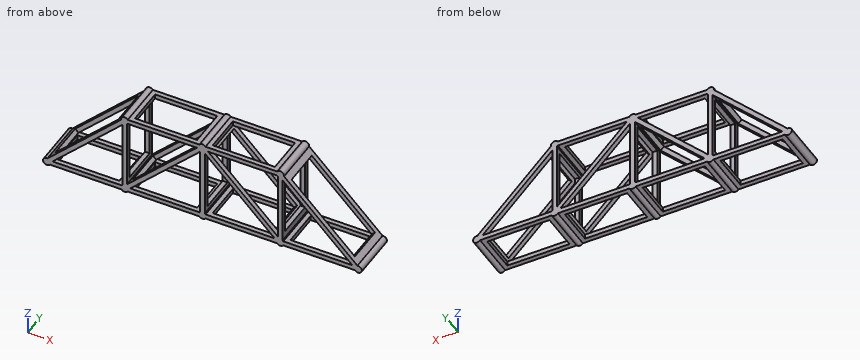
Autodesk Fusion 360 part; units mm, degrees
sketch "Sketch1" plane through (0, 0, 0) normal (0, 1, 0) x (1, 0, 0)
  circle A0 centre (-75, 0) radius 2.5
  line L0 (-75, 0) -> (25, 0) construction
  circle A1 centre (25, 0) radius 2.5
  line L1 (25, 0) -> (25, -50) construction
  line L2 (25, -50) -> (-25, -50) construction
  line L3 (-25, -50) -> (-75, 0) construction
  line L4 (25, -50) -> (-25, 0) construction
  line L5 (-25, -50) -> (-25, 0) construction
  circle A2 centre (-25, -50) radius 2.5
  circle A3 centre (25, -50) radius 2.5
  circle A4 centre (-25, 0) radius 2.5
  line L6 (-23.9393, -48.9393) -> (-73.9393, 1.0607)
  line L7 (-26.0607, -51.0607) -> (-76.0607, -1.0607)
  line L8 (25, -48.5) -> (-25, -48.5)
  line L9 (25, -51.5) -> (-25, -51.5)
  line L10 (23.5, 0) -> (23.5, -50)
  line L11 (26.5, 0) -> (26.5, -50)
  line L12 (23.9393, -51.0607) -> (-26.0607, -1.0607)
  line L13 (26.0607, -48.9393) -> (-23.9393, 1.0607)
  line L14 (-75, -1.5) -> (25, -1.5)
  line L15 (-75, 1.5) -> (25, 1.5)
  line L16 (-23.5, -50) -> (-23.5, 0)
  line L17 (-26.5, -50) -> (-26.5, 0)
  dimension "d1" = 5
  dimension "d2" = 5
  dimension "d3" = 5
  dimension "d4" = 5
  dimension "d5" = 5
  dimension "d6" = 1.5
  dimension "d7" = -1.5
  dimension "d8" = 1.5
  dimension "d9" = -1.5
  dimension "d10" = 1.5
  dimension "d11" = -1.5
  dimension "d12" = -1.5
  dimension "d13" = 1.5
  dimension "d14" = 1.5
  dimension "d15" = -1.5
  dimension "d16" = 1.5
  dimension "d17" = -1.5
extrude "Extrude1" add sketch "Sketch1" along normal blind 30 contours A0 | A0 A4 L6 L14 L15 | A0 L6 L14 | A0 A2 L6 L7 L14 L17 | A4 L14 L15 | A4 L15 | A2 L6 L8 | A1 A4 L13 L14 L15 | A4 L14 L17 | A2 A4 L6 L12 L16 L17 | A2 L6 L17 | A2 A3 L8 L9 L12 | A1 L10 L14 | A4 L12 L14 L17 | A2 L6 L8 L16 | A3 L8 L10 | A4 L13 L14 | A1 L10 L14 | A4 L12 L14 L16 | A4 L12 L16 | A2 L8 L16 | A3 L8 L12 | A3 A4 L8 L10 L12 L13 L14 L16 | A4 L14 L16 | A1 A3 L10 L11 L13 | A3 L8 L10 | A3 L10 L13
sketch "Sketch2" plane through (26.5, 0, 0) normal (1, 0, 0) x (0, 1, 0)
  line L0 (0, 48) -> (0, 2)
  line L1 (0, 2) -> (30, 2)
  line L2 (30, 2) -> (30, 48)
  line L3 (30, 48) -> (0, 48)
  line L4 (3, 45) -> (27, 45)
  line L5 (27, 45) -> (27, 5)
  line L6 (27, 5) -> (3, 5)
  line L7 (3, 5) -> (3, 45)
  dimension "d20" = 3
  dimension "d21" = 3
  dimension "d22" = 3
  dimension "d23" = 3
extrude "Extrude2" cut sketch "Sketch2" against normal blind 3 contours L4 L5 L6 L7
sketch "Sketch3" plane through (-11.4393, 0, 11.4393) normal (0.7071, 0, -0.7071) x (0, 1, 0)
  line L0 (0, 49.4117) -> (0, -14.0563)
  line L1 (0, -14.0563) -> (30, -14.0563)
  line L2 (30, -14.0563) -> (30, 49.4117)
  line L3 (30, 49.4117) -> (0, 49.4117)
  line L4 (3, 46.4117) -> (27, 46.4117)
  line L5 (27, 46.4117) -> (27, -11.0563)
  line L6 (3, -11.0563) -> (3, 46.4117)
  line L7 (3, -11.0563) -> (27, -11.0563)
  dimension "d27" = 3
  dimension "d28" = 3
  dimension "d29" = 3
  dimension "d31" = 3
extrude "Extrude3" cut sketch "Sketch3" against normal blind 3 contours L4 L5 L6 L7
sketch "Sketch4" plane through (-23.5, 0, 0) normal (1, 0, 0) x (0, 1, 0)
  line L0 (0, 48) -> (0, 3.6213)
  line L1 (0, 3.6213) -> (30, 3.6213)
  line L2 (30, 3.6213) -> (30, 48)
  line L3 (30, 48) -> (0, 48)
  line L4 (3, 45) -> (3, 6.6213)
  line L5 (3, 6.6213) -> (27, 6.6213)
  line L6 (27, 6.6213) -> (27, 45)
  line L7 (27, 45) -> (3, 45)
  dimension "d34" = 3
  dimension "d35" = 3
  dimension "d36" = 3
  dimension "d37" = 3
extrude "Extrude4" cut sketch "Sketch4" against normal blind 3 contours L4 L5 L6 L7
sketch "Sketch5" plane through (-36.4393, 0, 36.4393) normal (0.7071, 0, -0.7071) x (0, 1, 0)
  line L0 (0, 14.0563) -> (0, -49.4117)
  line L1 (0, -49.4117) -> (30, -49.4117)
  line L2 (30, -49.4117) -> (30, 14.0563)
  line L3 (30, 14.0563) -> (0, 14.0563)
  line L4 (3, 11.0563) -> (27, 11.0563)
  line L5 (27, 11.0563) -> (27, -46.4117)
  line L6 (3, -46.4117) -> (27, -46.4117)
  line L7 (3, 11.0563) -> (3, -46.4117)
  dimension "d41" = 3
  dimension "d42" = 3
  dimension "d43" = 3
  dimension "d44" = 3
extrude "Extrude5" cut sketch "Sketch5" against normal blind 3 contours L4 L5 L6 L7
ref_plane "WorkPlane1" through (25, 15, 24.1893) normal (-1, 0, 0) x (0, 0, 1)
sketch "Sketch6" plane through (0, 0, 51.5) normal (0, 0, 1) x (-1, 0, 0)
  line L0 (23, 0) -> (-23, 0)
  line L1 (-23, 0) -> (-23, -30)
  line L2 (-23, -30) -> (23, -30)
  line L3 (23, -30) -> (23, 0)
  line L4 (20, -27) -> (-20, -27)
  line L5 (-20, -27) -> (-20, -3)
  line L6 (-20, -3) -> (20, -3)
  line L7 (20, -3) -> (20, -27)
  dimension "d47" = 3
  dimension "d48" = 3
  dimension "d49" = 3
  dimension "d50" = 3
extrude "Extrude6" cut sketch "Sketch6" against normal blind 3 contours L4 L5 L6 L7
sketch "Sketch7" plane through (0, 0, -1.5) normal (0, 0, -1) x (1, 0, 0)
  line L0 (23, 0) -> (-23, 0)
  line L1 (-23, 0) -> (-23, -30)
  line L2 (-23, -30) -> (23, -30)
  line L3 (23, -30) -> (23, 0)
  line L4 (20, -27) -> (-20, -27)
  line L5 (-20, -27) -> (-20, -3)
  line L6 (-20, -3) -> (20, -3)
  line L7 (20, -3) -> (20, -27)
  dimension "d53" = 3
  dimension "d54" = 3
  dimension "d55" = 3
  dimension "d56" = 3
extrude "Extrude7" cut sketch "Sketch7" against normal blind 3 contours L4 L5 L6 L7
sketch "Sketch8" plane through (0, 0, -1.5) normal (0, 0, -1) x (1, 0, 0)
  line L0 (-27, 0) -> (-73, 0)
  line L1 (-73, 0) -> (-73, -30)
  line L2 (-73, -30) -> (-27, -30)
  line L3 (-27, -30) -> (-27, 0)
  line L4 (-30, -27) -> (-70, -27)
  line L5 (-70, -27) -> (-70, -3)
  line L6 (-70, -3) -> (-30, -3)
  line L7 (-30, -3) -> (-30, -27)
  dimension "d59" = 3
  dimension "d60" = 3
  dimension "d61" = 3
  dimension "d62" = 3
extrude "Extrude8" cut sketch "Sketch8" against normal blind 3 contours L4 L5 L6 L7
mirror "Mirror1" about plane through (25, 15, 24.1893) normal (-1, 0, 0) of bodies 1 merged
Work out the finished part from the listing and answer in its coordinate system (mm). Round coordinates to 2 decimals unless told otherwise and drop trailing zeros. Loops run counter-clockwise (first coordinate to the right, second up) from the corner with the lowest first, then second, coordinate; pieces in that order, holes last. Notation, with made-up numbers: (11.5, -38) - (66.5, -38) arc R18 cw to (66.5, -29) - close; hole circle Ø4 at (55.5, -40). An arc over 180 degrees is marked (long way). One line per item, written item: value.
Q1. Find section B-B on x = 38.5. Give the vertices of the cut face in (y, z), and give its area (3 significant figures).
Check values:
outline: (0, -1.5) - (3, -1.5) - (3, 1.5) - (0, 1.5) - close; (0, 34.38) - (3, 34.38) - (3, 38.62) - (0, 38.62) - close; (0, 48.5) - (3, 48.5) - (3, 51.5) - (0, 51.5) - close; (27, -1.5) - (30, -1.5) - (30, 1.5) - (27, 1.5) - close; (27, 34.38) - (30, 34.38) - (30, 38.62) - (27, 38.62) - close; (27, 48.5) - (30, 48.5) - (30, 51.5) - (27, 51.5) - close
area: 61.5 mm2
Q2. Find section C-C on y = 5.25. State how many separate pieces and enclosed holes the cut face has, and give its area (3 significant figures).
Check values:
separate pieces: 8
enclosed holes: 0
area: 403 mm2
Q3. Straight lines are drawn through the part: probe 1 along Y at (x, z) = (110, 16); probe 2 along X at (y, z) = (6.75, 47); probe 3 along Z at (x, y) = (60.5, 27.5). For each, find the intervals that lie inside material, in ascending order.
Check values:
probe 1: 0 to 3, 27 to 30
probe 2: -30.12 to -23.5, 19.88 to 30.12, 73.5 to 80.12
probe 3: -1.5 to 1.5, 12.38 to 16.62, 48.5 to 51.5
Q4. Find section A-A on x = -54.5. Give the vertices of the cut face in (y, z), and give its area (3 significant figures).
Check values:
outline: (0, -1.5) - (3, -1.5) - (3, 1.5) - (0, 1.5) - close; (0, 18.38) - (3, 18.38) - (3, 22.62) - (0, 22.62) - close; (27, -1.5) - (30, -1.5) - (30, 1.5) - (27, 1.5) - close; (27, 18.38) - (30, 18.38) - (30, 22.62) - (27, 22.62) - close
area: 43.5 mm2
Q5. Each of these flat-tipped pins is pushed along its axis until it touches: pin 1 Ø1.5 at (y, z) = (21.5, 4) entering from -X; pin 2 Ø15 at (x, y) = (105, 11.5) entering from +Z; pin 3 Ø12 at (x, y) = (-35, 15) entering from -Z; pin 4 Ø3.5 at (y, z) = (16.5, 50.5) entering from -X. Where does it stop, or does it pass through?
Check values:
pin 1: x = -73.87
pin 2: through
pin 3: z = -1.5
pin 4: x = -28.37
